Geometry check sheet. Reference: the model listing, model coordinates, mm. A direction names the side the tool comes from. Round coordinates to 2 decimals unless told otherwise and drop trailing zeros. Loops run counter-clockwise (first coordinate to the right, second up) from the corner with the lowest first, then second, coordinate; pieces in that order, holes last.
```python
from build123d import *
from OCP.BRepFilletAPI import BRepFilletAPI_MakeChamfer

# Parameters (mm, degrees)
SKETCH1_W           = 40
SKETCH1_H           = 40
BOSS_EXTRUDE1_DEPTH = 4
CUT_EXTRUDE1_REACH  = 30.566
SKETCH2_R           = 2.75
BOSS_EXTRUDE2_DEPTH = 6
CHAMFER1_SIZE       = 11
CHAMFER1_SIZE2      = 13.583868722
SKETCH4_R           = 2.6
CUT_EXTRUDE2_DEPTH  = 7
BOSS_EXTRUDE3_DEPTH = 2.75
CHAMFER2_SIZE       = 2
FILLET1_R           = 5


with BuildPart() as part:
    # Sketch1 → Boss-Extrude1 (new body)
    with BuildSketch(Plane.XY):
        Rectangle(SKETCH1_W, SKETCH1_H)
    extrude(amount=BOSS_EXTRUDE1_DEPTH)

    # Sketch2 → Cut-Extrude1 (cut, up to next)
    with BuildSketch(Plane.XY, mode=Mode.PRIVATE) as cut_extrude1_sk1:
        with Locations((-13, 13)):
            Circle(SKETCH2_R)
    cut_extrude1_tool1 = extrude(cut_extrude1_sk1.sketch, amount=CUT_EXTRUDE1_REACH, mode=Mode.PRIVATE) & part.part
    # Sketch2 → Cut-Extrude1 (cut, up to next)
    with BuildSketch(Plane.XY, mode=Mode.PRIVATE) as cut_extrude1_sk2:
        with Locations(Location((13, 13, 0), (0, 0, 180))):
            Circle(SKETCH2_R)
    cut_extrude1_tool2 = extrude(cut_extrude1_sk2.sketch, amount=CUT_EXTRUDE1_REACH, mode=Mode.PRIVATE) & part.part
    # Sketch2 → Cut-Extrude1 (cut, up to next)
    with BuildSketch(Plane.XY, mode=Mode.PRIVATE) as cut_extrude1_sk3:
        with Locations((13, -13)):
            Circle(SKETCH2_R)
    cut_extrude1_tool3 = extrude(cut_extrude1_sk3.sketch, amount=CUT_EXTRUDE1_REACH, mode=Mode.PRIVATE) & part.part
    # Sketch2 → Cut-Extrude1 (cut, up to next)
    with BuildSketch(Plane.XY, mode=Mode.PRIVATE) as cut_extrude1_sk4:
        with Locations(Location((-13, -13, 0), (0, 0, 180))):
            Circle(SKETCH2_R)
    cut_extrude1_tool4 = extrude(cut_extrude1_sk4.sketch, amount=CUT_EXTRUDE1_REACH, mode=Mode.PRIVATE) & part.part
    add(cut_extrude1_tool1.solids().sort_by_distance((-13, 13, 0))[0], mode=Mode.SUBTRACT)
    add(cut_extrude1_tool2.solids().sort_by_distance((13, 13, 0))[0], mode=Mode.SUBTRACT)
    add(cut_extrude1_tool3.solids().sort_by_distance((13, -13, 0))[0], mode=Mode.SUBTRACT)
    add(cut_extrude1_tool4.solids().sort_by_distance((-13, -13, 0))[0], mode=Mode.SUBTRACT)

    # Sketch3 → Boss-Extrude2 (add, symmetric)
    with BuildSketch(Plane(origin=(0, 0, 0), x_dir=(1, 0, 0), z_dir=(0, 1, 0))):
        with BuildLine():
            Line((-7, -4), (-7, -39))
            Line((-7, -39), (3, -39))
            Line((3, -39), (3, -31.952358141))
            ThreePointArc((3, -31.952358141), (-2.952358141, -22), (7, -16.047641859))
            Line((7, -16.047641859), (7, -4))
            Line((7, -4), (-7, -4))
        make_face()
    extrude(amount=BOSS_EXTRUDE2_DEPTH, both=True)

    # Chamfer1: one chamfer whose edges measure the first distance from different faces: ONE call of the kernel's chamfer builder (chamfer() names one face for all edges)
    chamfer1_edges_1 = [part.edges().sort_by_distance(p)[0] for p in [
        (0, -6, 4),
    ]]
    chamfer1_side_1 = [part.faces().sort_by_distance(p)[0] for p in [
        (6.623038464, -6, 10.02382093),
    ]]
    chamfer1_edges_2 = [part.edges().sort_by_distance(p)[0] for p in [
        (0, 6, 4),
    ]]
    chamfer1_side_2 = [part.faces().sort_by_distance(p)[0] for p in [
        (6.623038464, 6, 10.02382093),
    ]]
    chamfer1 = BRepFilletAPI_MakeChamfer(part.part.solid().wrapped)
    for e in chamfer1_edges_1:
        chamfer1.Add(CHAMFER1_SIZE, CHAMFER1_SIZE2, e.wrapped, chamfer1_side_1[0].wrapped)  # the first distance lies on this face
    for e in chamfer1_edges_2:
        chamfer1.Add(CHAMFER1_SIZE, CHAMFER1_SIZE2, e.wrapped, chamfer1_side_2[0].wrapped)  # the first distance lies on this face
    add(Compound.cast(chamfer1.Shape()), mode=Mode.REPLACE)

    # Sketch4 → Cut-Extrude2 (cut, symmetric)
    with BuildSketch(Plane(origin=(0, 0, 0), x_dir=(0, 0, -1), z_dir=(1, 0, 0))):
        with Locations((-13, 0)):
            Circle(SKETCH4_R)
        with Locations((-35, 0)):
            Circle(SKETCH4_R)
    extrude(amount=CUT_EXTRUDE2_DEPTH, both=True, mode=Mode.SUBTRACT)

    # Sketch5 → Boss-Extrude3 (add, symmetric)
    with BuildSketch(Plane(origin=(0, 0, 0), x_dir=(1, 0, 0), z_dir=(0, 1, 0))):
        with BuildLine():
            Line((7, -15.738644179), (7, -18.290140107))
            ThreePointArc((7, -18.290140107), (-0.709859893, -22), (3, -29.709859893))
            Line((3, -29.709859893), (3, -32.261355821))
            ThreePointArc((3, -32.261355821), (-3.261355821, -22), (7, -15.738644179))
        make_face()
    extrude(amount=BOSS_EXTRUDE3_DEPTH, both=True)

    # Chamfer2
    chamfer2_edges = [part.edges().sort_by_distance(p)[0] for p in [
        (7, 0, 4),
        (-7, 0, 4),
    ]]
    chamfer(chamfer2_edges, length=CHAMFER2_SIZE)

    # Fillet1
    fillet1_edges = [part.edges().sort_by_distance(p)[0] for p in [
        (20, -20, 2),
        (-20, -20, 2),
        (-20, 20, 2),
        (20, 20, 2),
    ]]
    fillet(fillet1_edges, radius=FILLET1_R)


solid = part.part
```
1) Sectioned sample at D-D, the plane x = 5. Record the cut outline in (y, z), then the cut area to 3 significant figures.
Report:
outline: (-20, 0) - (20, 0) - (20, 4) - (19.58, 4) - (6, 15) - (6, 15.8) - (2.75, 15.8) - (2.75, 17.95) - (-2.75, 17.95) - (-2.75, 15.8) - (-6, 15.8) - (-6, 15) - (-19.58, 4) - (-20, 4) - close; hole (-0.71, 15.5) arc R2.6 ccw (long way) to (0.71, 15.5) - close
area: 442 mm2
2) Sectioned sample at B-B, the plane x = -13. Record the cut outline in (y, z).
Report:
outline: (-20, 0) - (-15.75, 0) - (-15.75, 4) - (-20, 4) - close; (-10.25, 0) - (10.25, 0) - (10.25, 4) - (-10.25, 4) - close; (15.75, 0) - (20, 0) - (20, 4) - (15.75, 4) - close
3) Scan lines: line 1 along Y through (x, z) = (-13, 1); line 2 along Y through (x, z) = (-3.75, 35). Record each from-to range of solid material in increasing order.
Report:
line 1: y = -20 to -15.75, -10.25 to 10.25, 15.75 to 20
line 2: y = -6 to -2.6, 2.6 to 6
4) Sectioned sample at C-C, the plane y = -14. Record the cut outline in (x, z), then the cut area to 3 significant figures.
Report:
outline: (-20, 0) - (-15.56, 0) - (-15.56, 4) - (-20, 4) - close; (-10.44, 0) - (10.44, 0) - (10.44, 4) - (9, 4) - (7, 6) - (7, 8.52) - (-7, 8.52) - (-7, 6) - (-9, 4) - (-10.44, 4) - close; (15.56, 0) - (20, 0) - (20, 4) - (15.56, 4) - close
area: 186 mm2
5) Access from +Z, -Z, +X, -X, +Y, -Y to the whole of each face (thin tool, end or side, straight path). Record for faces 4 (the face through (5, 0, 15.5)), 5 (the face through (-7, 0, 19)), 6 (the face through (-3, 6, 27)).
Report:
face 4: none
face 5: +Z, -X, +Y, -Y
face 6: +Z, +X, -X, +Y
6) Gauge pin test, flat ends, axial feed: pin 1 (8 mm diameter, centred on y = 7, z = 32.5, fed in from +X); pin 2 (2 mm diameter, centred on x = 5, z = 10, fed in from -Y); pin 3 (3 mm diameter, centred on x = 3, z = 21, fed in from +Y); pin 4 (5 mm diameter, centred on x = 3.5, y = -12, fed in from +Z). Record the tip position at first contact, or that the pin passes through.
Report:
pin 1: stops at x = 3
pin 2: stops at y = -13.41
pin 3: passes through
pin 4: stops at z = 12.17
7) Sectioned sample at A-A, the plane z = 35. Record the cut outline in (x, y).
Report:
outline: (-7, -6) - (3, -6) - (3, -2.6) - (-7, -2.6) - close; (-7, 2.6) - (3, 2.6) - (3, 6) - (-7, 6) - close
8) Mould release check, pull along Z, two halves, no side actions. Record for faces 1 (the face through (-20, 0, 2)), 2 (the face through (-8, 0, 5)), 3 (the face through (-3, 4.4, 22.2)): +Z half, -Z half, draft (parallel to the pull), parting line (faces both ways), or undercut.
Report:
face 1: draft
face 2: +Z half
face 3: undercut
